Input: part model. Units: mm. Frame: model coordinates. A direction names the side the tool comes from. Coordinates: 2 decimals unless noted, no trailing zeros. Loops run counter-clockwise (first coordinate to the right, second up) from the corner with the lowest first, then second, coordinate; pieces in that order, holes last. Notation, with made-up numbers: (25.5, 69) -> (32.5, 69) arc R21 cw to (32.5, 99) -> close; hole circle Ø7 at (39.5, -1.5). An arc over 180 degrees is marked (long way). Answer as a JSON object with one key per item and string values.
from build123d import *

# Parameters (mm, degrees)
F0_W     = 66.675
F0_H     = 88.9
F1_DEPTH = 44.45
F2_T     = -1.27
F4_DEPTH = 5.08
F5_W     = 66.675
F5_H     = 12.7
F6_DEPTH = 0.5
F7_W     = 66.675
F7_H     = 12.6965791702
F8_DEPTH = 0.5
F9_DEPTH = 25.4


with BuildPart() as f1:
    # F0 (on Top) → F1 (new body)
    with BuildSketch(Plane.XY):
        with Locations((-1.1231470853, 10.8568438743)):
            Rectangle(F0_W, F0_H)
    extrude(amount=F1_DEPTH)

    # F2
    f2_openings = [f1.faces().sort_by_distance(p)[0] for p in [
        (-1.123147, 10.856844, 44.45),
    ]]
    offset(amount=F2_T, openings=f2_openings)

    # F3 (on face) → F4 (join)
    with BuildSketch(Plane.XY.offset(1.27)):
        Polygon((30.9443529147, 41.3368438743), (28.4043529147, 41.3368438743), (28.4043529147, -0.1921561257), (28.4043529147, -3.3671561257), (28.4043529147, -9.4631561257), (30.9443529147, -9.4631561257), align=None)
        Polygon((-30.6506470853, 41.3368438743), (-33.1906470853, 41.3368438743), (-33.1906470853, -9.4631561257), (-30.6506470853, -9.4631561257), (-30.6506470853, -3.3671561257), (-30.6506470853, -0.1921561257), align=None)
    extrude(amount=F4_DEPTH)

    # F5 (on face) → F6 (join)
    with BuildSketch(Plane(origin=(0, 55.3068438743, 0), x_dir=(-1, 0, 0), z_dir=(0, 1, 0))):
        with Locations((1.1231470853, 38.1)):
            Rectangle(F5_W, F5_H)
    extrude(amount=F6_DEPTH)

    # F7 (on face) → F8 (join)
    with BuildSketch(Plane.XZ.offset(33.5931561257)):
        with Locations((-1.1231470853, 38.1017104149)):
            Rectangle(F7_W, F7_H)
    extrude(amount=F8_DEPTH)

    # F3 (on face) → F9 (cut)
    with BuildSketch(Plane.XY.offset(1.27)):
        Polygon((-33.1906470853, 54.0368438743), (-33.1906470853, 41.3368438743), (-30.6506470853, 41.3368438743), (28.4043529147, 41.3368438743), (30.9443529147, 41.3368438743), (30.9443529147, 54.0368438743), align=None)
    extrude(amount=-F9_DEPTH, mode=Mode.SUBTRACT)


solid = f1.part
1. Mould query, pull axis X, two halves, no side actions, for faces 5 (the face through (32.214, 11, 22)), 6 (the face through (28.404, 16, 4)), 7 (the face through (-33.4, 31, 44.45)). Classes: pulls with the +X half, pulls with the -X half, needs draft (parallel to the pull), parting line crosses it, or undercut.
Reply:
{"face 5": "pulls with the +X half", "face 6": "undercut", "face 7": "needs draft"}
2. Section query B-B (x = -19). Return loops of the section in (y, z).
Reply:
{"outline": "(-34.09, 31.75) -> (-33.59, 31.75) -> (-33.59, 0) -> (41.34, 0) -> (41.34, 1.27) -> (-32.32, 1.27) -> (-32.32, 44.45) -> (-34.09, 44.45) -> close; (54.04, 0) -> (55.31, 0) -> (55.31, 31.75) -> (55.81, 31.75) -> (55.81, 44.45) -> (54.04, 44.45) -> close"}
3. Section query C-C (z = 40). Return loops of the section in (x, y).
Reply:
{"outline": "(-34.46, -34.09) -> (32.21, -34.09) -> (32.21, 55.81) -> (-34.46, 55.81) -> close; hole (-33.19, -32.32) -> (30.94, -32.32) -> (30.94, 54.04) -> (-33.19, 54.04) -> close"}
4. Line query: line 1 along X through (y, z) = (-23, 7); line 2 along Y through (x, z) = (-31, 40); line 3 along Y through (x, z) = (0, 3.5). Output: solid intervals per line, ascending.
Reply:
{"line 1": "x = -34.46 to -33.19, 30.94 to 32.21", "line 2": "y = -34.09 to -32.32, 54.04 to 55.81", "line 3": "y = -33.59 to -32.32, 54.04 to 55.31"}
5. Section query A-A (y = 43). Return loops of the section in (x, z), plus the area to 3 significant figures.
Reply:
{"outline": "(-34.46, 0) -> (-33.19, 0) -> (-33.19, 44.45) -> (-34.46, 44.45) -> close; (30.94, 0) -> (32.21, 0) -> (32.21, 44.45) -> (30.94, 44.45) -> close", "area": "113 mm2"}
6. Section query D-D (y = 33.5). Return loops of the section in (x, z).
Reply:
{"outline": "(-34.46, 0) -> (32.21, 0) -> (32.21, 44.45) -> (30.94, 44.45) -> (30.94, 6.35) -> (28.4, 6.35) -> (28.4, 1.27) -> (-30.65, 1.27) -> (-30.65, 6.35) -> (-33.19, 6.35) -> (-33.19, 44.45) -> (-34.46, 44.45) -> close"}
7. Access query for faces 1 (the face through (-2, -33.593, 16)), 2 (the face through (-33.191, 10, 22)), 3 (the face through (-2, 55.307, 16)), 4 (the face through (-2, 54.037, 22)). Directions: +Z, -Z, +X, -X, +Y, -Y. A direction counts if a zero-diameter tool reaches every point of the face in a straight line with its end or side. Return the directions, or none.
Reply:
{"face 1": "-Z, +X, -X, -Y", "face 2": "+Z", "face 3": "-Z, +X, -X, +Y", "face 4": "+Z, -Z"}
8. Pin query (flat end, axial travel): P1, Ø3, axis at x = -12, z = 6.5, coming from the +Y side; P2, Ø2, axis at x = -32, z = 4, coming from the -Y side; P3, Ø0.6, axis at x = 12.5, y = -34, coming from the -Z side. Return the tip coordinate at first contact, or that it passes through.
Reply:
{"P1": "stops at y = 55.31", "P2": "stops at y = -33.59", "P3": "stops at z = 31.75"}
